```python
from build123d import *

# Parameters (mm, degrees)
SKETCH1_R           = 5
SKETCH1_R_2         = 1.905
BOSS_EXTRUDE1_DEPTH = 10
FILLET1_R           = 2.54
SCALE1_SCALE        = 0.66


with BuildPart() as part:
    # Sketch1 → Boss-Extrude1 (new body)
    with BuildSketch(Plane(origin=(0, 0, 0), x_dir=(1, 0, 0), z_dir=(0, 1, 0))):
        with BuildLine():
            Line((-36.007707984, -8.333333333), (6.325625349, -36.414089892))
            ThreePointArc((6.325625349, -36.414089892), (18.236180718, -35.778760148), (21.066179973, -24.191867669))
            Line((21.066179973, -24.191867669), (9.21284664, 3.888888889))
            ThreePointArc((9.21284664, 3.888888889), (5.527707984, 8.333333333), (0, 10))
            Line((0, 10), (-30.48, 10))
            ThreePointArc((-30.48, 10), (-40.054271078, 2.886751346), (-36.007707984, -8.333333333))
        make_face()
        with Locations((-30.48, 0)):
            Circle(SKETCH1_R, mode=Mode.SUBTRACT)
        Circle(SKETCH1_R, mode=Mode.SUBTRACT)
        with Locations((11.853333333, -28.080756558)):
            Circle(SKETCH1_R, mode=Mode.SUBTRACT)
        with Locations((10.953276102, -13.297076469)):
            Circle(SKETCH1_R_2, mode=Mode.SUBTRACT)
    extrude(amount=BOSS_EXTRUDE1_DEPTH)

    # Fillet1
    fillet1_edges = [part.edges().sort_by_distance(p)[0] for p in [
        (18.236180718, 10, 35.778760148),
        (15.139513307, 10, 10.15148939),
        (5.527707984, 10, -8.333333333),
        (-15.24, 10, -10),
        (-40.054271078, 10, -2.886751346),
        (-15.24, 0, -10),
        (5.527707984, 0, -8.333333333),
        (15.139513307, 0, 10.15148939),
        (-14.841041317, 10, 22.373711613),
        (18.236180718, 0, 35.778760148),
        (-14.841041317, 0, 22.373711613),
        (-40.054271078, 0, -2.886751346),
    ]]
    fillet(fillet1_edges, radius=FILLET1_R)


with BuildPart() as part_1:
    # Scale1: scaled about (-6.985968974, 5, 10.314628386)
    add(part.part.scale(SCALE1_SCALE).moved(Location((-2.375229451, 1.7, 3.506973651))))


solid = part_1.part
```
Design review of the part built by this model. Coordinates are the model's own, in mm. Give positions to 0.01 mm unless a question says otherwise; leave off trailing zeros. Order: outer loops, then holes, each group sorted by start corner. A loop starts at its lowest first (then second) coordinate and runs counter-clockwise, first axis right, second up. Notation, with made-up numbers: (46.25, -9.75) -> (91.25, -9.75) arc R13 ccw to (91.25, 0.25) -> close; hole circle Ø6 at (-35, -7.75). An arc over 180 degrees is marked (long way). Write item = value, one per line. Start each with the question number.
(1) For pin 1 (3 mm diameter, centred on x = 4.85, z = 12.28, fed in from -Y); pin 2 (3 mm diameter, centred on y = 4.5, z = 12, fed in from +X); pin 3 (1.5 mm diameter, centred on y = 5.5, z = 7, fed in from +X), all flat-tipped, find the tip position at first contact; note any pin that passes through.
(2) We need section A-A on y = 5. Write out the cut boundary in (x, z).
(3) Mouldability with a two-part tool opening along X and no side actions: class faces 1 (the face through (-28.776, 4.977, 1.489)), 2 (the face through (4.69, 4.954, 11.036)), 3 (the face through (7.122, 7.796, 10.263)) as +X half, -X half, draft (parallel to the pull), parting line (faces both ways), or undercut.
(4) We need section C-C on y = 7.5. Write out the cut boundary in (x, z), plus the area to 3 significant figures.
(5) We need section B-B on x = 5. State how many separate pieces and enclosed holes the cut face has, plus the area to 3 significant figures.
(6) To check wall thickness, follow line 1 along X through (y, z) = (4.5, 5.5); line 2 along Z through (x, y) = (4, 5.25); line 3 along Z through (x, y) = (-5, 2.75). State the ranges of each line that lie inside material, in increasing order.
Numbers:
q1.pin_1 = 1.7
q1.pin_2 = 9.01
q1.pin_3 = 6.58
q2.outline = (-26.14, 9.01) arc R6.6 ccw to (-22.49, -3.09) -> (-2.38, -3.09) arc R6.6 ccw to (3.71, 0.94) -> (11.53, 19.47) arc R6.6 ccw to (1.8, 27.54) -> close; hole circle Ø6.6 at (-22.49, 3.51); hole circle Ø6.6 at (-2.38, 3.51); hole circle Ø6.6 at (5.45, 22.04); hole circle Ø2.51 at (4.85, 12.28)
q3.face_1 = -X half
q3.face_2 = undercut
q3.face_3 = +X half
q4.outline = (-26, 8.8) arc R6.35 ccw to (-22.49, -2.85) -> (-2.38, -2.85) arc R6.35 ccw to (3.48, 1.04) -> (11.3, 19.57) arc R6.35 ccw to (1.94, 27.33) -> close; hole circle Ø6.6 at (-22.49, 3.51); hole circle Ø6.6 at (-2.38, 3.51); hole circle Ø6.6 at (5.45, 22.04); hole circle Ø2.51 at (4.85, 12.28)
q4.area = 674 mm^2
q5.separate_pieces = 3
q5.enclosed_holes = 0
q5.area = 98.5 mm^2
q6.line_1 = -28.78 to -25.12, -19.86 to -5.01, 0.25 to 5.63
q6.line_2 = 1.64 to 11.36, 13.21 to 19.07, 25.01 to 28.48
q6.line_3 = -2.97 to 1.51, 5.51 to 22.88
